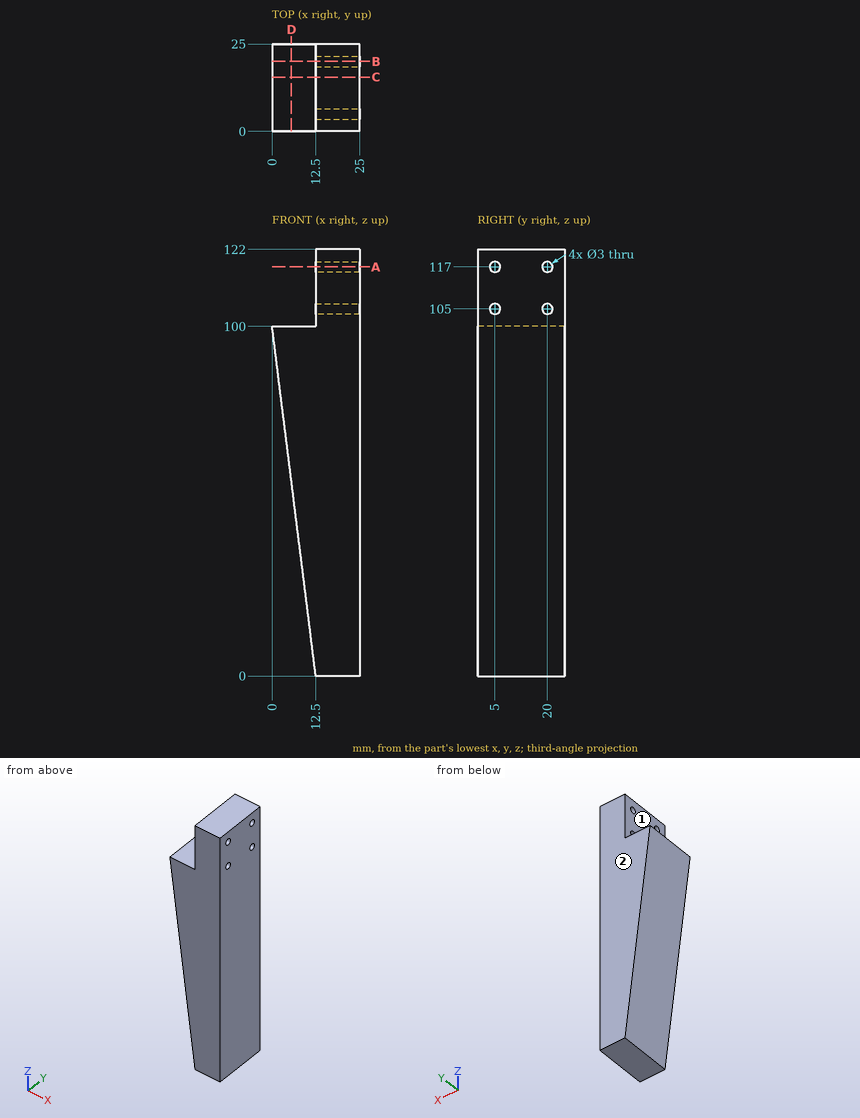
The drawing under review shows one solid part. Ordinate dimensions are in mm from its lowest x, y, z. A direction names the side the tool comes from. Round coordinates to 2 decimals unless told otherwise and drop trailing zeros. Write each loop counter-clockwise with the first axis right and the second up, starting at its lowest first coordinate (ties: lowest second). Pieces come first, ordered by that corner, then holes. Notation, with made-up numbers: (-25, 79) -> (-12, 79) arc R34 cw to (-12, 117) -> close; hole circle Ø11 at (57, 28). An arc over 180 degrees is marked (long way). One line per question, with ' | ' between items. Start each with the question number.
(1) Add section D-D, the plane x = 5.5. Write out the cut boundary in (y, z), plus the area to 3 significant figures.
(2) Add section B-B, the plane y = 20. Write out the cut boundary in (x, z).
(3) Add section C-C, the plane y = 15.5. Write out the cut boundary in (x, z), plus the area to 3 significant figures.
(4) Tool access review of the marked faces 1 and 2: name each direction out of +Z, -Z, +X, -X, +Y, -Y from which nothing blocks a thin tool from reaching the whole face with its end or side.
(5) Add section A-A, the plane z = 117. Write out the cut boundary in (x, y).
(6) Insertion check: P1, Ø3.5, axis at y = 5, z = 117, coming from the -X side; P2, Ø12, axis at x = 5.5, y = 20.5, coming from the +Z side. Each pin has a flat end and moves straight along its axis. Give the tip position at first contact, or say it passes through.
(7) For line 1 along Y through (x, z) = (15.75, 105); line 2 along X through (y, z) = (15, 110); line 3 along Z through (x, y) = (17, 6.25), list the stretches that pass through material, from the lowest coordinate up. Write a range as from..to.
Answer list:
1) outline: (0, 56) -> (25, 56) -> (25, 100) -> (0, 100) -> close | area: 1,100 mm²
2) outline: (0, 100) -> (12.5, 0) -> (25, 0) -> (25, 103.5) -> (12.5, 103.5) -> (12.5, 100) -> close; (12.5, 106.5) -> (25, 106.5) -> (25, 115.5) -> (12.5, 115.5) -> close; (12.5, 118.5) -> (25, 118.5) -> (25, 122) -> (12.5, 122) -> close
3) outline: (0, 100) -> (12.5, 0) -> (25, 0) -> (25, 122) -> (12.5, 122) -> (12.5, 100) -> close | area: 2,150 mm²
4) face 1: +Z, -X, +Y, -Y | face 2: +Z, -Z, +X, -X, +Y
5) outline: (12.5, 0) -> (25, 0) -> (25, 3.5) -> (12.5, 3.5) -> close; (12.5, 6.5) -> (25, 6.5) -> (25, 18.5) -> (12.5, 18.5) -> close; (12.5, 21.5) -> (25, 21.5) -> (25, 25) -> (12.5, 25) -> close
6) P1: x = 12.5 | P2: z = 100
7) line 1: 0..3.5, 6.5..18.5, 21.5..25 | line 2: 12.5..25 | line 3: 0..104.17, 105.83..116.17, 117.83..122
